The listing builds one solid part. Answer for the finished solid, in the listing's coordinates (mm). Round coordinates to 2 decimals unless told otherwise and drop trailing zeros. Write each loop counter-clockwise with the first axis right and the second up, starting at its lowest first coordinate (ties: lowest second). Pieces come first, ordered by that corner, then holes. Notation, with made-up numbers: (25.25, 35.25) - (72.25, 35.25) arc R16 cw to (72.25, 42.25) - close; hole circle Ø4 at (23.25, 24). An arc over 180 degrees is marked (long way). Answer in a Markdown table with one row per item.
from build123d import *

# Parameters (mm, degrees)
F1_DEPTH       = 9.128125
F3_D           = 2.032
F3_CSINK_D     = 3.175
F3_CSINK_ANGLE = 82
F5_D           = 2.54
F5_CSINK_D     = 6.35
F5_CSINK_ANGLE = 82


with BuildPart() as f1:
    # F0 (on Top) → F1 (new body, symmetric)
    with BuildSketch(Plane.XY):
        Polygon((-16.14385, 0), (-38.262192, 22.486981), (-38.262192, 0), align=None)
    extrude(amount=F1_DEPTH, both=True)

    # F3 (through all)
    with Locations(Plane(origin=(-8.205336, -8.070822, 0), x_dir=(-0.701239, 0.712926, 0), z_dir=(0.712926, 0.701239, 0))):
        with Locations((17.670697, -5.159375), (17.670697, 5.159375)):
            CounterSinkHole(F3_D / 2, F3_CSINK_D / 2, counter_sink_angle=F3_CSINK_ANGLE)

    # F5 (through all)
    with Locations(Plane.XZ):
        with Locations((-33.499692, 0)):
            CounterSinkHole(F5_D / 2, F5_CSINK_D / 2, counter_sink_angle=F5_CSINK_ANGLE)


solid = f1.part
(1) Section C-C (y = 14) is taken. Give the vertices of the cut face in (x, z), and give its area (3 significant figures).
Checked values:
| item | result |
|---|---|
| outline | (-38.26, -9.13) - (-29.91, -9.13) - (-29.91, 9.13) - (-38.26, 9.13) - close; hole circle Ø2.54 at (-33.5, 0) |
| area | 147 mm2 |
(2) Find the intervals of material crossed by line 1 (X direction, y = 13, z = 0); line 2 (X direction, y = 14.75, z = 0); line 3 (X direction, y = 10.5, z = -1.5), in increasing order.
Checked values:
| item | result |
|---|---|
| line 1 | x = -38.26 to -34.77, -32.23 to -28.93 |
| line 2 | x = -38.26 to -34.77, -32.23 to -30.65 |
| line 3 | x = -38.26 to -26.47 |
(3) Flat-ended cylindrical pins translate along their axes: pin 1 (4 mm diameter, centred on x = -28.5, z = 0, fed in from +Y); pin 2 (1 mm diameter, centred on y = 5, z = -5, fed in from +X); pin 3 (2 mm diameter, centred on x = -31.5, z = -7, fed in from -Y); pin 4 (1 mm diameter, centred on x = -26.5, y = 12, fed in from -Z). Find the tip coordinate at first contact, or state that the pin passes through.
Checked values:
| item | result |
|---|---|
| pin 1 | stops at y = 14.6 |
| pin 2 | stops at x = -21.62 |
| pin 3 | stops at y = 0 |
| pin 4 | passes through |
(4) Section B-B (z = -8) is taken. Give the vertices of the cut face in (x, y), and give its area (3 significant figures).
Checked values:
| item | result |
|---|---|
| outline | (-38.26, 0) - (-16.14, 0) - (-38.26, 22.49) - close |
| area | 249 mm2 |
(5) Section D-D (y = 16.5) is taken. Give the vertices of the cut face in (x, z), and give its area (3 significant figures).
Checked values:
| item | result |
|---|---|
| outline | (-38.26, -9.13) - (-32.37, -9.13) - (-32.37, -0.59) arc R1.27 cw (long way) to (-32.37, 0.59) - (-32.37, 9.13) - (-38.26, 9.13) - close |
| area | 103 mm2 |
(6) Section A-A (z = 0) is taken. Give the vertices of the cut face in (x, y).
Checked values:
| item | result |
|---|---|
| outline | (-38.26, 0) - (-36.67, 0) - (-34.77, 2.19) - (-34.77, 18.94) - (-38.26, 22.49) - close; (-32.23, 2.19) - (-30.32, 0) - (-16.14, 0) - (-32.23, 16.35) - close |
(7) For a pull along X with two mould halves and no side action, classify faces 1 (the flat face through (-27.05, 11.09, 0.13)), 2 (the cylindrical face through (-23.7, 2.9, -5.1)), 3 (the flat face through (-27, 0, 0)) as pulls with the +X half, pulls with the -X half, needs draft (parallel to the pull), parting line crosses it, or undercut.
Checked values:
| item | result |
|---|---|
| face 1 | pulls with the +X half |
| face 2 | undercut |
| face 3 | needs draft |
